Study the drawing (mm; zero at the part's minimum x, y, z) and answer. A direction names the side the tool comes from. Give positions to 0.01 mm unless a question says otherwise; leave off trailing zeros. Loops run counter-clockwise (first coordinate to the right, second up) from the corner with the lowest first, then second, coordinate; pieces in that order, holes last. Notation, with made-up numbers: M 22,17.25 L 40,17.25 A17 ccw 40,41.25 Z; hole C 43,-27.75 d11. An arc over 180 degrees is marked long. Return JSON: item names as keys, results as strings.
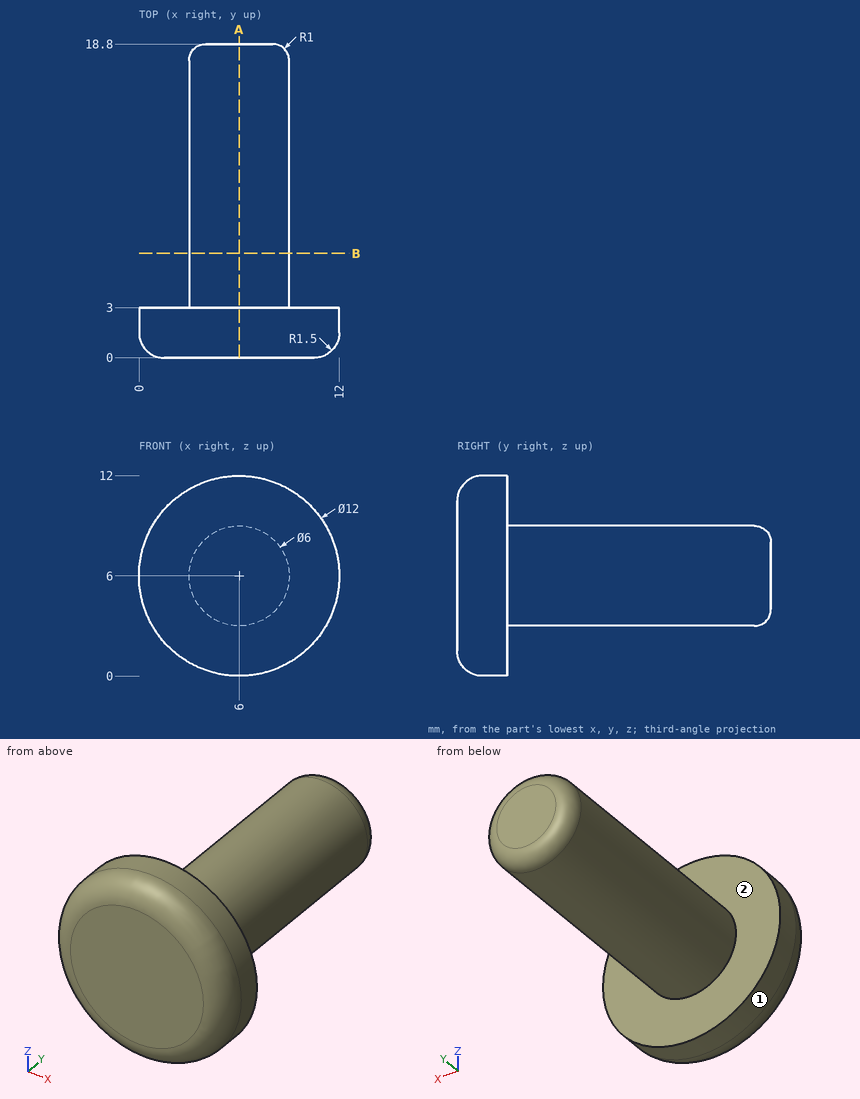
(1) A tool of negligible diameter and unlimited length cuts with its end or side. For the marked faces 1 and 2, from which of +Z, -Z, +X, -X, +Y, -Y can it reach the whole face along a straight path? Write none if from no direction.
Values follow:
{"face 1": "+Y, -Y", "face 2": "+Y"}
(2) The part is cut by section B-B (y = 6.25). Determine the outline of the cut face in (x, z), and give its area (3 significant figures).
Values follow:
{"outline": "C 6,6 d6", "area": "28.3 mm²"}
(3) Straight lines are drawn through the part: line 1 along Y through (x, z) = (9.25, 4.75); line 2 along Z through (x, y) = (6, 15.25); line 3 along X through (y, z) = (3.5, 4.75). For each, find the intervals that lie inside material, in ascending order.
Values follow:
{"line 1": "0 to 3", "line 2": "3 to 9", "line 3": "3.27 to 8.73"}
(4) Given pin 1 (4 mm diameter, centred on x = 5, y = 4, fed in from +Z); pin 2 (2 mm diameter, centred on y = 3.5, z = 8.5, fed in from -X); pin 3 (3 mm diameter, centred on x = 6.5, y = 12.5, fed in from +Z); pin 4 (1.5 mm diameter, centred on y = 4, z = 7.5, fed in from +X), each flat-ended and moving along its own axis, determine where each tip first touches the part or whether it passes through.
Values follow:
{"pin 1": "z = 12", "pin 2": "x = 0.23", "pin 3": "z = 9", "pin 4": "x = 8.9"}
(5) The part is cut by section A-A (x = 6). Determine the outline of the cut face in (y, z).
Values follow:
{"outline": "M 0,1.5 A1.5 ccw 1.5,0 L 3,0 L 3,3 L 17.8,3 A1 ccw 18.8,4 L 18.8,8 A1 ccw 17.8,9 L 3,9 L 3,12 L 1.5,12 A1.5 ccw 0,10.5 Z"}
